```python
from build123d import *
from build123d.topology import SkipClean

# Parameters (mm, degrees)
SKETCH1_R                        = 2.1
FINGER_BASE_1_DEPTH              = 6
SKETCH2_W                        = 16
SKETCH2_H                        = 2
FLEXURE_JOINT_BASE_DEPTH         = 13
SKETCH3_W                        = 8
SKETCH3_H                        = 2
PULLEY_HOUSING_DEPTH             = 3
M3_NUT_DEPTH                     = 2
SKETCH5_R                        = 1.725
M3_HOLE_DEPTH                    = 3
SKETCH9_W                        = 2
SKETCH9_H                        = 2
SUPPORT_FLEXURE_JOINT_BASE_DEPTH = 4.5
SKETCH10_R                       = 0.725
HOLE_FOR_STICHING_DEPTH          = 22.391190815
CUT_EXTRUDE1_DEPTH               = 32.362649657
CUT_EXTRUDE1_DEPTH_BACK          = 32.362649657


with BuildPart() as part:
    # Sketch1 → Finger Base 1 (new, symmetric)
    with BuildSketch(Plane.XY):
        Polygon((0, 8.221825407), (7.778174593, 16), (9.889087297, 16), (9.889087297, 18), (17.889087297, 18), (17.889087297, 16), (19.8, 16), (19.8, 0), (0, 0), align=None)
        with Locations((9.151471863, 6)):
            Circle(SKETCH1_R, mode=Mode.SUBTRACT)
    extrude(amount=FINGER_BASE_1_DEPTH, both=True)

    # Sketch2 → Flexure Joint Base (add)
    with BuildSketch(Plane(origin=(-4.110912703, 4.110912703, 0), x_dir=(0, 0, 1), z_dir=(-0.7071067811865462, 0.707106781186549, 0))):
        with Locations((0, 8.313708499)):
            Rectangle(SKETCH2_W, SKETCH2_H)
    extrude(amount=FLEXURE_JOINT_BASE_DEPTH)

    # Sketch3 → Pulley Housing (cut, symmetric)
    with SkipClean():  # the faces are left unmerged after this step: merging them gives an invalid solid
        with BuildSketch(Plane.XY):
            with BuildLine():
                ThreePointArc((7.054725188, 6.116847687), (7.62579494, 4.556978889), (9.151471863, 3.9))
                Line((9.151471863, 3.9), (9.151471863, 0))
                Line((9.151471863, 0), (19.8, 0))
                Line((19.8, 0), (19.8, 11))
                Line((19.8, 11), (9.889087297, 11))
                Line((9.889087297, 11), (9.889087297, 16))
                Line((9.889087297, 16), (7.778174593, 16))
                Line((7.778174593, 16), (2.474873734, 10.696699141))
                Line((2.474873734, 10.696699141), (7.054725188, 6.116847687))
            make_face()
            with Locations((13.889087297, 17)):
                Rectangle(SKETCH3_W, SKETCH3_H)
        extrude(amount=PULLEY_HOUSING_DEPTH, both=True, mode=Mode.SUBTRACT)
    add(part.part.scale(1), mode=Mode.REPLACE)  # the faces are merged on a copy

    # Sketch4 → M3 Nut (cut)
    with BuildSketch(Plane.XZ.offset(-11)):
        Polygon((10.598190762, 0), (12.243639029, -2.85), (15.534535564, -2.85), (17.179983831, 0), (15.534535564, 2.85), (12.243639029, 2.85), align=None)
    extrude(amount=-M3_NUT_DEPTH, mode=Mode.SUBTRACT)

    # Sketch5 → M3 Hole (cut)
    with BuildSketch(Plane.XZ.offset(-13)):
        with Locations(Location((13.889087297, 0, 0), (0, 0, 270))):
            Circle(SKETCH5_R)
    extrude(amount=-M3_HOLE_DEPTH, mode=Mode.SUBTRACT)

    # Sketch9 → Support Flexure Joint Base (add)
    with BuildSketch(Plane(origin=(-4.110912703, 4.110912703, 0), x_dir=(0, 0, -1), z_dir=(0.7071067811865462, -0.7071067811865488, 0))):
        with Locations((-7, 8.313708499)):
            Rectangle(SKETCH9_W, SKETCH9_H)
        with Locations((7, 8.313708499)):
            Rectangle(SKETCH9_W, SKETCH9_H)
    extrude(amount=SUPPORT_FLEXURE_JOINT_BASE_DEPTH)

    # Sketch10 → Hole For Stiching (cut, through all)
    with BuildSketch(Plane(origin=(6.585786438, 6.585786438, 0), x_dir=(0.7071067811865462, -0.707106781186549, 0), z_dir=(0.707106781186549, 0.7071067811865462, 0))):
        with Locations(Location((-16.313708499, -5.5, 0), (0, 0, 180))):
            Circle(SKETCH10_R)
        with Locations(Location((-10.813708499, -5.5, 0), (0, 0, 180))):
            Circle(SKETCH10_R)
        with Locations(Location((-10.813708499, 5.5, 0), (0, 0, 180))):
            Circle(SKETCH10_R)
        with Locations(Location((-16.313708499, 5.5, 0), (0, 0, 180))):
            Circle(SKETCH10_R)
    extrude(amount=-HOLE_FOR_STICHING_DEPTH, mode=Mode.SUBTRACT)

    # Sketch11 → Cut-Extrude1 (cut, two sides: drawn at the far end of the back side and taken through both)
    with BuildSketch(Plane.XY.offset(6).offset(-CUT_EXTRUDE1_DEPTH_BACK)):
        Polygon((-30.849385448, 48.263599011), (4.596194078, 12.818019485), (6.01040764, 11.403805922), (7.424621202, 12.818019485), (6.01040764, 14.232233047), (-29.435171886, 49.677812573), (-100.326330938, 120.568971625), (-101.7405445, 119.154758062), align=None)
    extrude(amount=CUT_EXTRUDE1_DEPTH + CUT_EXTRUDE1_DEPTH_BACK, mode=Mode.SUBTRACT)


solid = part.part
```
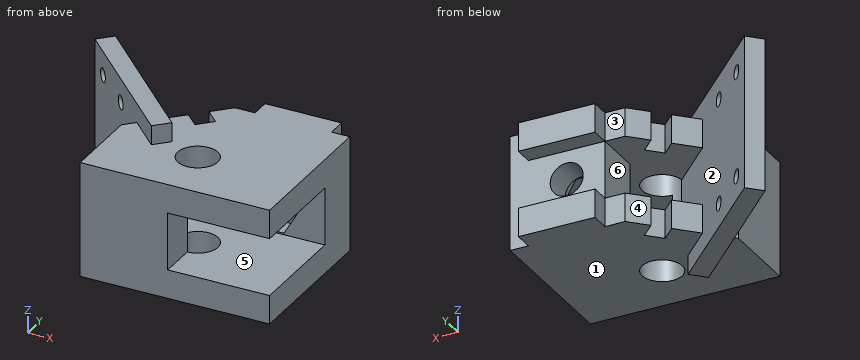
For this review, take the finished solid that the model builds, in its own axes (mm). Face numbers are marked on the shaded views. A direction names the side the tool comes from. Coordinates: 2 decimals unless noted, no trailing zeros. Loops run counter-clockwise (first coordinate to the right, second up) from the corner with the lowest first, then second, coordinate; pieces in that order, holes last.
1. Add section D-D, the plane x = 8.75. Give the boundary of the cut face in (y, z).
2. Add section A-A, the plane z = -0.5. Give the boundary of the cut face in (x, y).
3. Add section C-C, the plane z = 2.5. Give the boundary of the cut face in (x, y).
4. Add section B-B, the plane x = 14.25. Give the boundary of the cut face in (y, z), then the cut area to 3 significant figures.
5. Mouldability with a two-part tool opening along Z and no side actions: class the marked faces 1, 2 and 3 as +Z half, -Z half, draft (parallel to the pull), parting line (faces both ways), or undercut.
6. For line 1 (Z direction, x = 7.5, y = 13.25); line 2 (X direction, y = 14.1, z = 0); line 3 (X direction, y = 15.3, z = 0), list the stretches that pass through material, from the lowest coordinate up.
7. Insertion check: P1, Ø1.5, axis at x = 12.5, z = 4.5, coming from the +Y side; P2, Ø5.5, axis at y = 14.5, z = 0.5, coming from the -X side; P3, Ø8, axis at x = 1.5, z = 3, coming from the +Y side. Each pin has a flat end and moves straight along its axis. Give the tip position at first contact, or say it passes through.
8. For the marked faces 4, 5 and 6, list the 3-axis set-ups (+Z, -Z, +X, -X, +Y, -Y) from which the entire face can be reached by the end or side of a thin tool; tool diameter is ignored.
Result:
1. outline: (0, -6) - (3.94, -6) - (3.94, 6) - (0, 6) - close; (8.06, -6) - (16, -6) - (16, -3) - (8.06, -3) - close; (8.06, 3) - (16, 3) - (16, 6) - (8.06, 6) - close
2. outline: (-8.13, 18.47) - (1.06, 9.28) - (0, 8.22) - (0, 0) - (9.15, 0) - (9.15, 3.9) arc R2.1 cw to (7.05, 6.12) - (-6.72, 19.89) - close; (9.89, 11) - (10.89, 11) - (10.89, 13) - (12.24, 13) - (12.24, 16) - (9.89, 16) - close; (15.54, 13) - (16.89, 13) - (16.89, 11) - (19.8, 11) - (19.8, 16) - (15.54, 16) - close
3. outline: (-8.13, 18.47) - (1.06, 9.28) - (0, 8.22) - (0, 0) - (9.15, 0) - (9.15, 3.9) arc R2.1 cw to (7.05, 6.12) - (-6.72, 19.89) - close; (9.89, 11) - (12.04, 11) - (12.04, 13) - (15.74, 13) - (15.74, 11) - (19.8, 11) - (19.8, 16) - (9.89, 16) - close
4. outline: (0, -6) - (18, -6) - (18, -3) - (16, -3) - (16, -1.69) - (13, -1.69) - (13, -2.85) - (11, -2.85) - (11, -3) - (0, -3) - close; (0, 3) - (11, 3) - (11, 2.85) - (13, 2.85) - (13, 1.69) - (16, 1.69) - (16, 3) - (18, 3) - (18, 6) - (0, 6) - close
4. area: 116 mm2
5. face 1: -Z half
5. face 2: undercut
5. face 3: draft
6. line 1: z = -6 to -3, 3 to 6
6. line 2: x = -3.76 to -0.93, 9.89 to 12.16, 15.61 to 19.8
6. line 3: x = -4.96 to -2.13, 9.89 to 12.16, 15.61 to 19.8
7. P1: stops at y = 18
7. P2: stops at x = -6.91
7. P3: stops at y = 15.67
8. face 4: +Z, -Z, +Y
8. face 5: none
8. face 6: +Y, -Y
